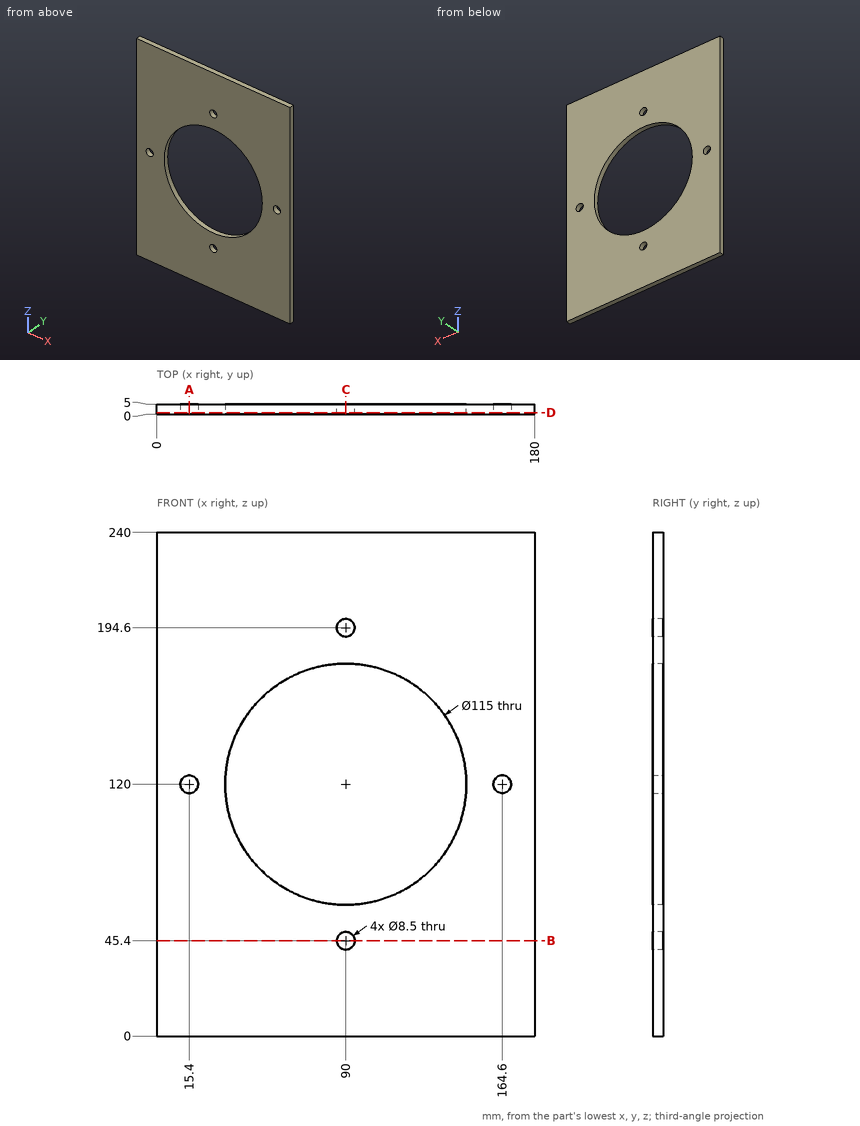
Geometry: see drawing. Coordinates: mm, zero at the bounding-box minimum. Round coordinates to 2 decimals unless told otherwise and drop trailing zeros. Loops run counter-clockwise (first coordinate to the right, second up) from the corner with the lowest first, then second, coordinate; pieces in that order, holes last. Notation, with made-up numbers: (-34, 28) - (2, 28) arc R19 cw to (2, 52) - close; hole circle Ø10 at (-39.5, -21.75). An arc over 180 degrees is marked (long way). Write item = value, one per line. Start each with the question number.
(1) Section query A-A, the plane x = 15.4. Output: boundary loops of the cut face in (y, z), plus the area to 3 significant figures.
(2) Ray query, line 1 along Z through (x, y) = (90, 1.2); line 2 along X through (y, z) = (3.55, 120); line 3 along Z through (x, y) = (92, 3.3). Return the intervals inside material, ascending. Write a range as from..to.
(3) Pin query (flat end, axial travel): pin 1 (11 mm diameter, centred on x = 15.4, z = 120, fed in from +Y). Return the tip coordinate at first contact, or that it passes through.
(4) Section query C-C, the plane x = 90. Output: boundary loops of the cut face in (y, z).
(5) Section query B-B, the plane z = 45.4. Output: boundary loops of the cut face in (x, y).
(6) Section query D-D, the plane y = 0.9. Output: boundary loops of the cut face in (x, z), plus the area to 3 significant figures.
Conclusion:
q1.outline = (0, 0) - (5, 0) - (5, 115.75) - (0, 115.75) - close; (0, 124.25) - (5, 124.25) - (5, 240) - (0, 240) - close
q1.area = 1,160 mm2
q2.line_1 = 0..41.15, 49.65..62.5, 177.5..190.35, 198.85..240
q2.line_2 = 0..11.15, 19.65..32.5, 147.5..160.35, 168.85..180
q2.line_3 = 0..41.65, 49.15..62.53, 177.47..190.85, 198.35..240
q3.pin_1 = 5
q4.outline = (0, 0) - (5, 0) - (5, 41.15) - (0, 41.15) - close; (0, 49.65) - (5, 49.65) - (5, 62.5) - (0, 62.5) - close; (0, 177.5) - (5, 177.5) - (5, 190.35) - (0, 190.35) - close; (0, 198.85) - (5, 198.85) - (5, 240) - (0, 240) - close
q5.outline = (0, 0) - (85.75, 0) - (85.75, 5) - (0, 5) - close; (94.25, 0) - (180, 0) - (180, 5) - (94.25, 5) - close
q6.outline = (0, 0) - (180, 0) - (180, 240) - (0, 240) - close; hole circle Ø8.5 at (15.4, 120); hole circle Ø115 at (90, 120); hole circle Ø8.5 at (90, 45.4); hole circle Ø8.5 at (90, 194.6); hole circle Ø8.5 at (164.6, 120)
q6.area = 32,600 mm2
